Check sheet for the drawn part. Datum: minimum x, y, z corner. Units: mm. Round coordinates to 2 decimals unless told otherwise and drop trailing zeros. Write each loop counter-clockwise with the first axis right and the second up, starting at its lowest first coordinate (ties: lowest second). Pieces come first, ordered by that corner, then holes. Notation, with made-up numbers: (61.5, -38) - (110.5, -38) arc R16 cw to (110.5, -24) - close; hole circle Ø11 at (57, 74). An arc over 180 degrees is marked (long way). Return JSON: item names as keys, results as strings. Group by question number.
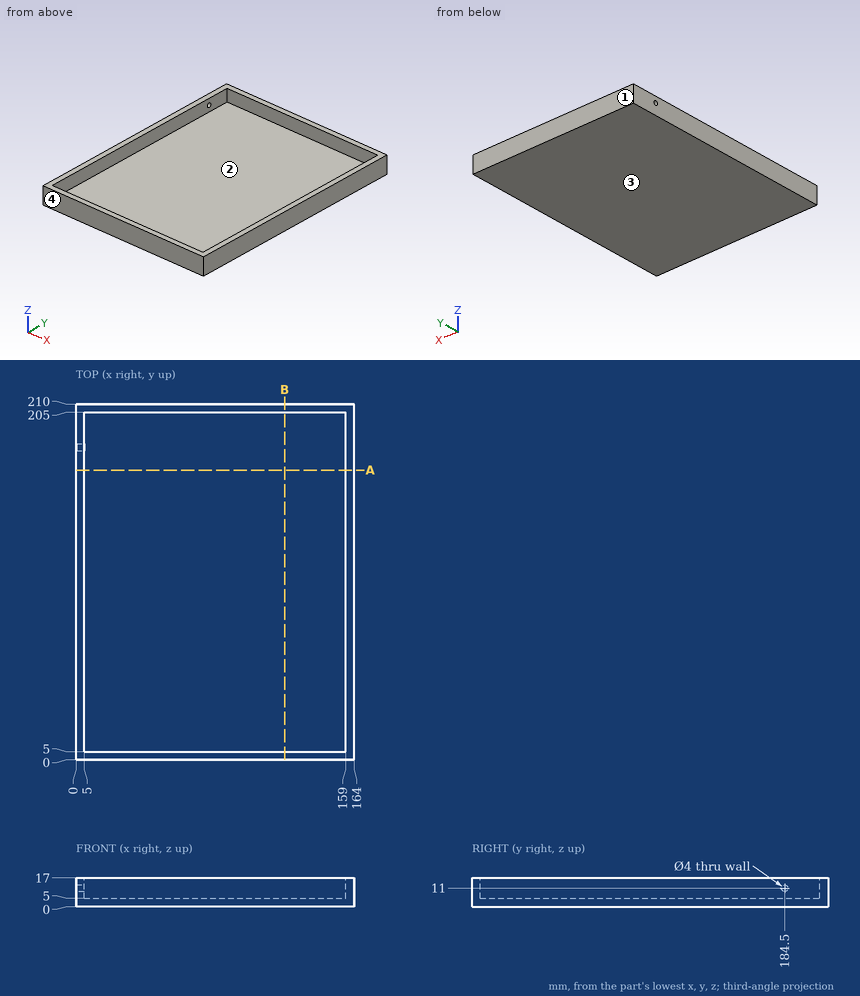
1. Depth check by flat-ended pin: pin 1 Ø1.5 at (x, z) = (130.5, 4.5) entering from -Y. Enter the tip coordinate at first touch or a pass-through.
2. Section check B-B (x = 123). Enter the section's corners in (y, z).
3. Section check A-A (y = 171). Enter the section's corners in (x, z).
4. Material ranges on line 1 along X through (y, z) = (116, 12); line 2 along Y through (x, z) = (12, 14.75); line 3 along Z through (x, y) = (2, 184.5), recorded low to high.
5. Mould release check, pull along Y, two halves, no side actions. Record for the marked faces 1, 2, 3 and 4: pulls with the +Y half, pulls with the -Y half, needs draft (parallel to the pull), parting line crosses it, or undercut.
Result sheet:
{
 "1": {"pin 1": "stops at y = 0"},
 "2": {"outline": "(0, 0) - (210, 0) - (210, 17) - (205, 17) - (205, 5) - (5, 5) - (5, 17) - (0, 17) - close"},
 "3": {"outline": "(0, 0) - (164, 0) - (164, 17) - (159, 17) - (159, 5) - (5, 5) - (5, 17) - (0, 17) - close"},
 "4": {"line 1": "x = 0 to 5, 159 to 164", "line 2": "y = 0 to 5, 205 to 210", "line 3": "z = 0 to 9, 13 to 17"},
 "5": {"face 1": "pulls with the +Y half", "face 2": "undercut", "face 3": "needs draft", "face 4": "pulls with the -Y half"}
}
